```python
from build123d import *

# Parameters (mm, degrees)
SKETCH1_R           = 17.5
BOSS_EXTRUDE1_DEPTH = 3.5
SKETCH1_3_R         = 1.75
CUT_EXTRUDE1_DEPTH  = 3.5


with BuildPart() as part:
    # Sketch1 → Boss-Extrude1 (new body)
    with BuildSketch(Plane(origin=(0, 0, 0), x_dir=(1, 0, 0), z_dir=(0, 1, 0))):
        Circle(SKETCH1_R)
    extrude(amount=BOSS_EXTRUDE1_DEPTH)

    # Sketch1<3> → Cut-Extrude1 (cut)
    with BuildSketch(Plane(origin=(0, 0, 0), x_dir=(1, 0, 0), z_dir=(0, 1, 0))):
        Circle(SKETCH1_3_R)
        with Locations((0, 12.5)):
            Circle(SKETCH1_3_R)
        with Locations((-12.5, 0)):
            Circle(SKETCH1_3_R)
        with Locations((0, -12.5)):
            Circle(SKETCH1_3_R)
        with Locations((12.5, 0)):
            Circle(SKETCH1_3_R)
    extrude(amount=CUT_EXTRUDE1_DEPTH, mode=Mode.SUBTRACT)


solid = part.part
```
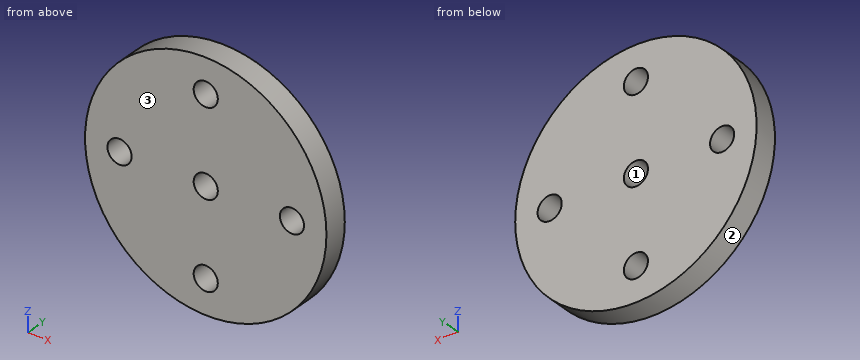
Read the model definition and answer for the solid it produces. Units are mm, in the model's axes. Face numbers are marked on the shaded views. Coordinates: 2 decimals unless noted, no trailing zeros. Write each loop counter-clockwise with the first axis right and the second up, starting at its lowest first coordinate (ties: lowest second). Pieces come first, ordered by that corner, then holes. Notation, with made-up numbers: (67, 20) -> (98, 20) arc R22 ccw to (98, 28) -> close; hole circle Ø2 at (-4, 27). An arc over 180 degrees is marked (long way). Answer as a JSON object with one key per item and string values.
Q1. The part is cut by section B-B on y = 2.1. Give the vertices of the cut face in (x, z), then the cut area to 3 significant figures.
The answers:
{"outline": "circle Ø35 at (0, 0); hole circle Ø3.5 at (-12.5, 0); hole circle Ø3.5 at (0, -12.5); hole circle Ø3.5 at (0, 0); hole circle Ø3.5 at (0, 12.5); hole circle Ø3.5 at (12.5, 0)", "area": "914 mm2"}
Q2. A flat-ended cylindrical pin translates along its axis: pin 1 Ø1 at (x, y) = (13, 3) entering from -Z. Find the tip coordinate at first contact, or state that the pin passes through.
The answers:
{"pin 1": "stops at z = -12.25"}
Q3. Determine the mould class of the marked faces 1, 2 and 3 for opening direction Z: pulls with the +Z half, pulls with the -Z half, needs draft (parallel to the pull), parting line crosses it, or undercut.
The answers:
{"face 1": "undercut", "face 2": "parting line crosses it", "face 3": "needs draft"}
Q4. The part is cut by section A-A on z = 0. Give the vertices of the cut face in (x, y), then the cut area to 4 significant figures.
The answers:
{"outline": "(-17.5, 0) -> (-14.25, 0) -> (-14.25, 3.5) -> (-17.5, 3.5) -> close; (-10.75, 0) -> (-1.75, 0) -> (-1.75, 3.5) -> (-10.75, 3.5) -> close; (1.75, 0) -> (10.75, 0) -> (10.75, 3.5) -> (1.75, 3.5) -> close; (14.25, 0) -> (17.5, 0) -> (17.5, 3.5) -> (14.25, 3.5) -> close", "area": "85.75 mm2"}
Q5. The part is cut by section D-D on z = -12.5. Give the vertices of the cut face in (x, y), then the cut area to 3 significant figures.
The answers:
{"outline": "(-12.25, 0) -> (-1.75, 0) -> (-1.75, 3.5) -> (-12.25, 3.5) -> close; (1.75, 0) -> (12.25, 0) -> (12.25, 3.5) -> (1.75, 3.5) -> close", "area": "73.5 mm2"}
Q6. The part is cut by section C-C on x = -11.5. Give the vertices of the cut face in (y, z), then the cut area to 3 significant figures.
The answers:
{"outline": "(0, -13.19) -> (3.5, -13.19) -> (3.5, -1.44) -> (0, -1.44) -> close; (0, 1.44) -> (3.5, 1.44) -> (3.5, 13.19) -> (0, 13.19) -> close", "area": "82.3 mm2"}
Q7. Consider line 1 (Z direction, x = 0, y = 2.6); line 2 (Z direction, x = 1.5, y = 2.2). Determine where each line is inside the solid, lowest interval first. Write a range as [from, to].
The answers:
{"line 1": "z = [-17.5, -14.25], [-10.75, -1.75], [1.75, 10.75], [14.25, 17.5]", "line 2": "z = [-17.44, -13.4], [-11.6, -0.9], [0.9, 11.6], [13.4, 17.44]"}
